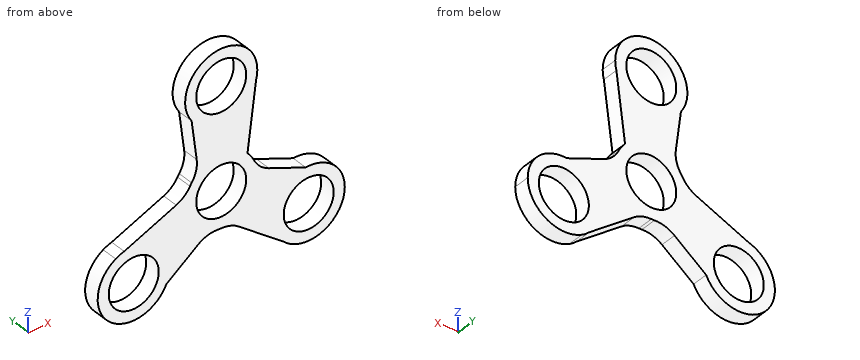
from build123d import *

# Parameters (mm, degrees)
F0_R     = 11
F1_DEPTH = 7


with BuildPart() as f1:
    # F0 (on Front) → F1 (new body)
    with BuildSketch(Plane.XZ):
        with BuildLine():
            ThreePointArc((-10.218251, -18.367249), (-6.0466, -16.265091), (-1.397113, -15.813403))
            ThreePointArc((-1.397113, -15.813403), (-0.720579, -15.858638), (-0.04273, -15.874942))
            ThreePointArc((-0.04273, -15.874942), (4.004964, -16.548747), (7.626532, -18.478019))
            Line((7.626532, -18.478019), (27.331615, -33.512077))
            ThreePointArc((27.331615, -33.512077), (23.570998, -16.812529), (37.162239, -6.406025))
            Line((37.162239, -6.406025), (21.01563, 0.33436))
            ThreePointArc((21.01563, 0.33436), (17.109282, 2.896038), (14.393365, 6.696766))
            ThreePointArc((14.393365, 6.696766), (13.14047, 8.907506), (11.550893, 10.890019))
            Line((11.550893, 10.890019), (15.356507, 40.42591))
            ThreePointArc((15.356507, 40.42591), (2.774582, 28.819347), (-13.033335, 35.386457))
            Line((-13.033335, 35.386457), (-10.797377, 18.03289))
            ThreePointArc((-10.797377, 18.03289), (-11.062681, 13.369055), (-12.996251, 9.116638))
            ThreePointArc((-12.996251, 9.116638), (-13.373693, 8.553359), (-13.726738, 7.974477))
            ThreePointArc((-13.726738, 7.974477), (-16.334117, 4.805974), (-19.8157, 2.634241))
            Line((-19.8157, 2.634241), (-42.688118, -6.913832))
            ThreePointArc((-42.688118, -6.913832), (-28.86552, -9.603907), (-22.619828, -22.225002))
            ThreePointArc((-22.619828, -22.225002), (-23.001689, -25.685967), (-24.128902, -28.980429))
            Line((-24.128902, -28.980429), (-10.218251, -18.367249))
        make_face()
        Circle(F0_R, mode=Mode.SUBTRACT)
        with BuildLine():
            ThreePointArc((-46.432329, -8.476849), (-49.23868, -33.911972), (-24.128902, -28.980429))
            ThreePointArc((-24.128902, -28.980429), (-23.001689, -25.685967), (-22.619828, -22.225002))
            ThreePointArc((-22.619828, -22.225002), (-28.86552, -9.603907), (-42.688118, -6.913832))
            Line((-42.688118, -6.913832), (-46.432329, -8.476849))
        make_face()
        with Locations((-38.494828, -22.225002)):
            Circle(F0_R, mode=Mode.SUBTRACT)
        with BuildLine():
            ThreePointArc((37.162239, -6.406025), (23.570998, -16.812529), (27.331615, -33.512077))
            Line((27.331615, -33.512077), (30.557333, -35.97315))
            ThreePointArc((30.557333, -35.97315), (46.432333, -35.973148), (54.369832, -22.224996))
            ThreePointArc((54.369832, -22.224996), (49.238684, -10.538026), (37.162239, -6.406025))
        make_face()
        with Locations((38.494832, -22.224996)):
            Circle(F0_R, mode=Mode.SUBTRACT)
        with BuildLine():
            Line((30.557333, -35.97315), (27.331615, -33.512077))
            ThreePointArc((27.331615, -33.512077), (28.865525, -34.846092), (30.557333, -35.97315))
        make_face()
        with BuildLine():
            ThreePointArc((-42.688118, -6.913832), (-44.610364, -7.575229), (-46.432329, -8.476849))
            Line((-46.432329, -8.476849), (-42.688118, -6.913832))
        make_face()
        with BuildLine():
            Line((15.875, 44.45), (15.356507, 40.42591))
            ThreePointArc((15.356507, 40.42591), (15.744843, 42.421322), (15.875, 44.45))
        make_face()
        with BuildLine():
            ThreePointArc((-13.033335, 35.386457), (2.774582, 28.819347), (15.356507, 40.42591))
            Line((15.356507, 40.42591), (15.875, 44.45))
            ThreePointArc((15.875, 44.45), (-4.749286, 59.597934), (-13.033335, 35.386457))
        make_face()
        with Locations((0, 44.45)):
            Circle(F0_R, mode=Mode.SUBTRACT)
    extrude(amount=F1_DEPTH)


solid = f1.part
Model file for the job. Use its own axes, mm. Round coordinates to 2 decimals unless told otherwise and drop trailing zeros. Loops run counter-clockwise (first coordinate to the right, second up) from the corner with the lowest first, then second, coordinate; pieces in that order, holes last. Notation, with made-up numbers: (9.25, 13.5) - (54.25, 13.5) arc R17 ccw to (54.25, 23.5) - close; hole circle Ø4 at (6.25, 28). An arc over 180 degrees is marked (long way). Write each question's results on one line, items separated by ' | '.
(1) Pin check, flat tips, straight feed: pin 1 (1.5 mm diameter, centred on y = -2, z = -17, fed in from +X); pin 2 (3 mm diameter, centred on y = -3.5, z = -24, fed in from -X); pin 3 (20 mm diameter, centred on x = 0, z = 0, fed in from +Y); pin 4 (4 mm diameter, centred on y = -3.5, z = 45, fed in from -X) (3 decimals). Stop position of each tip, or through.
Answer below:
pin 1: stops at x = 53.73 | pin 2: stops at x = -54.37 | pin 3: passes through | pin 4: stops at x = -15.875
(2) Wall check: L1, parallel to Z at x = 0, y = -3.75 (3 decimals); L2, parallel to X at y = -4, z = -21.5; L3, parallel to Z at x = 38, y = -1.5. Give the ranges that are in metal, low to high.
Answer below:
L1: z = -15.875 to -11, 11 to 33.45, 55.45 to 60.325 | L2: x = -54.35 to -49.47, -27.52 to -14.32, 11.59 to 27.52, 49.47 to 54.35 | L3: z = -38.09 to -33.21, -11.24 to -6.36
(3) Saw through at C-C, the plane x = 13. List the corners of the cut face in (y, z), then the cut area to 3 significant figures.
Answer below:
outline: (-7, -22.58) - (0, -22.58) - (0, 9.11) - (-7, 9.11) - close; (-7, 22.14) - (0, 22.14) - (0, 53.56) - (-7, 53.56) - close | area: 442 mm^2
(4) Saw through at B-B, the plane x = -36. List the corners of the cut face in (y, z), then the cut area to 3 significant figures.
Answer below:
outline: (-7, -37.9) - (0, -37.9) - (0, -32.94) - (-7, -32.94) - close; (-7, -11.51) - (0, -11.51) - (0, -4.12) - (-7, -4.12) - close | area: 86.5 mm^2
(5) Saw through at A-A, the plane y = -4.5. Count the separate pieces of the cut face and the enclosed holes in it, then the cut area to 3 significant figures.
Answer below:
separate pieces: 1 | enclosed holes: 4 | area: 2,870 mm^2
